Can you work these out from the model? Positions are in its coordinate system, mm. A direction names the side the tool comes from. Round coordinates to 2 decimals unless told otherwise and drop trailing zeros. Loops run counter-clockwise (first coordinate to the right, second up) from the corner with the lowest first, then second, coordinate; pieces in that order, holes last.
Autodesk Inventor part; units mm, degrees
ref_plane "YZ Plane" through (0, 0, 0) normal (1, 0, 0) x (0, 1, 0)
ref_plane "XZ Plane" through (0, 0, 0) normal (0, 1, 0) x (-1, 0, 0)
ref_plane "XY Plane" through (0, 0, 0) normal (0, 0, 1) x (1, 0, 0)
sketch "Sketch1" plane through (0, 0, 0) normal (0, 1, 0) x (-1, 0, 0)
  line L0 (10, -10) -> (-10, -10)
  line L1 (-10, -10) -> (-10, 10)
  line L2 (-10, 10) -> (10, 10)
  line L3 (10, 10) -> (10, -10)
  line L4 (10, -10) -> (-10, 10) construction
  line L5 (-10, -10) -> (10, 10) construction
  point P0 (0, 0)
  dimension "d0" = 20
  dimension "d1" = 20
extrude "Extrusion1" add sketch "Sketch1" along normal blind 700
sketch "Sketch2" plane through (0, 0, 0) normal (0, -1, 0) x (1, 0, 0)
  line L0 (-200, -10) -> (200, -10)
  line L1 (200, -10) -> (200, 10)
  line L2 (200, 10) -> (-200, 10)
  line L3 (-200, 10) -> (-200, -10)
  line L4 (-200, -10) -> (200, 10) construction
  line L5 (200, -10) -> (-200, 10) construction
  point P0 (0, 0)
  dimension "d4" = 400
  dimension "d5" = 20
extrude "Extrusion2" add sketch "Sketch2" along normal blind 20
sketch "Sketch3" plane through (0, -20, 0) normal (0, -1, 0) x (1, 0, 0)
  line L0 (-200, 10) -> (-200, -10)
  line L1 (-200, -10) -> (200, -10)
  line L2 (200, -10) -> (200, 10)
  line L3 (200, 10) -> (-200, 10)
  line L4 (0, 0) -> (0, -200)
  line L5 (10, 0) -> (-10, 0)
  line L6 (-10, 0) -> (-10, -200)
  line L7 (-10, -200) -> (10, -200)
  line L8 (10, -200) -> (10, 0)
  line L9 (10, 0) -> (-10, -200) construction
  line L10 (-10, 0) -> (10, -200) construction
  point P0 (0, -100)
  point P1 (10, -10)
  point P2 (-10, -10)
  dimension "d8" = 200
  dimension "d9" = 20
  dimension "d10" = 200
extrude "Extrusion3" add sketch "Sketch3" against normal blind 20 contours L1 L4 L7 L6 | L1 L8 L7 L4
properties part number "leg_sim_stand"
(1) For faces 1 (the flat face through (104, -10, -10)), 2 (the flat face through (10, 345, 0)), 3 (the flat face through (-10, -10, -104)), 4 (the flat face through (0, 0, -104)), which set-ups out of +Z, -Z, +X, -X, +Y, -Y let a thin tool reach every point of the face, with its end or its side?
Worked answers:
face 1: -Z, +X, +Y, -Y
face 2: +Z, -Z, +X, +Y
face 3: -Z, -X, +Y, -Y
face 4: -Z, +X, -X, +Y
(2) Will these pins go through, and if not, where does the flat tip stop? P1, Ø6, axis at x = -62, y = -8.5, coming from the -Z side; P2, Ø10, axis at y = 233, z = -2, coming from the +X side; P3, Ø10, axis at x = 96.5, z = 1.5, coming from the +Y side.
Worked answers:
P1: stops at z = -10
P2: stops at x = 10
P3: stops at y = 0
(3) If I drill on line 1 (Y direction, x = 99.5, z = -2), over which ranges is the centre line in solid material (lowest first)?
Worked answers:
line 1: y = -20 to 0
(4) If we section it at A-A, the plane x = -26.5: List the corners of the cut face in (y, z) for me.
Worked answers:
outline: (-20, -10) - (0, -10) - (0, 10) - (-20, 10) - close
(5) If we section it at B-B, the plane y = 202: List the corners of the cut face in (x, z) for me, then the cut area to 3 significant figures.
Worked answers:
outline: (-10, -10) - (10, -10) - (10, 10) - (-10, 10) - close
area: 400 mm2
